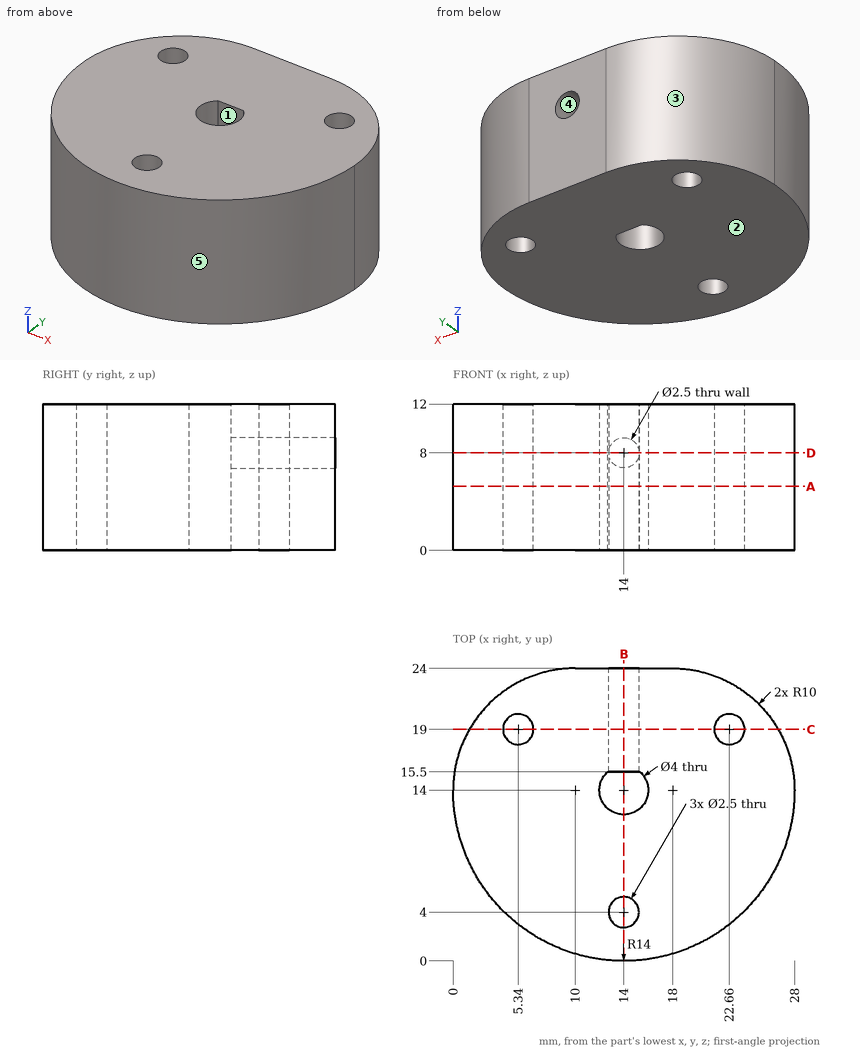
The drawing under review shows one solid part. Ordinate dimensions are in mm from its lowest x, y, z. A direction names the side the tool comes from. Give positions to 0.01 mm unless a question says otherwise; leave off trailing zeros. Order: outer loops, then holes, each group sorted by start corner. A loop starts at its lowest first (then second) coordinate and runs counter-clockwise, first axis right, second up. Notation, with made-up numbers: M 82.25,68 L 107.25,68 A22 cw 107.25,96 Z; hole C -8,32 d5. An arc over 180 degrees is marked long. Answer in a Markdown table with one row per item. Add a question column.
1. Machinability: for the marked faces 4 and 5, which of the approach directions +Z, -Z, +X, -X, +Y, -Y give a long, thin tool a straight path to every point of the face, cutting with its end or side? Answer none if there is none.
2. To check wall thickness, follow line 1 along X through (y, z) = (18, 3.5) (1 decimal); line 2 along Z through (x, y) = (14, 18); line 3 along Y through (x, z) = (4.5, 7) (1 decimal). State the ranges of each line that lie inside material, in increasing order.
3. Add section A-A on z = 5.25. State the section outline as (x, y) points, plus the area to 3 significant figures.
4. Add section C-C on y = 19. State the section outline as (x, z) points, plus the area to 3 significant figures.
5. Add section D-D on z = 8. State the section outline as (x, y) points.
6. For pin 1 Ø1.5 at (x, z) = (22, 7.5) entering from -Y; pin 2 Ø6 at (x, z) = (5.5, 8) entering from -Y (1 decimal); pin 3 Ø2 at (y, z) = (19, 3.5) entering from +X (1 decimal), all flat-tipped, find the tip position at first contact; note any pin that passes through.
7. Add section B-B on x = 14. State the section outline as (y, z) points.
8. Mouldability with a two-part tool opening along Y and no side actions: class the marked faces 1, 2 and 3 as released by +Y, released by -Y, zero draft, split by the parting line, or undercut.
The answers:
| question | item | result |
|---|---|---|
| 1 | face 4 | +Y |
| 1 | face 5 | +Z, -Z, -Y |
| 2 | line 1 | 0.8 to 4.6, 6.1 to 21.9, 23.4 to 27.2 |
| 2 | line 2 | 0 to 6.75, 9.25 to 12 |
| 2 | line 3 | 3.7 to 18.1, 19.9 to 22.4 |
| 3 | outline | M 0,14 A14 ccw 28,14 A10 ccw 18,24 L 10,24 A10 ccw Z; hole C 5.34,19 d2.5; hole M 12.68,15.5 A2 ccw long 15.32,15.5 Z; hole C 14,4 d2.5; hole C 22.66,19 d2.5 |
| 3 | area | 519 mm2 |
| 4 | outline | M 1.34,0 L 4.09,0 L 4.09,12 L 1.34,12 Z; M 6.59,0 L 21.41,0 L 21.41,12 L 6.59,12 Z; M 23.91,0 L 26.66,0 L 26.66,12 L 23.91,12 Z; hole C 14,8 d2.5 |
| 4 | area | 239 mm2 |
| 5 | outline | M 0,14 A14 ccw 28,14 A10 ccw 18,24 L 15.25,24 L 15.25,15.5 L 15.32,15.5 A2 cw long 12.68,15.5 L 12.75,15.5 L 12.75,24 L 10,24 A10 ccw Z; hole C 5.34,19 d2.5; hole C 14,4 d2.5; hole C 22.66,19 d2.5 |
| 6 | pin 1 | y = 2.02 |
| 6 | pin 2 | y = 1.1 |
| 6 | pin 3 | x = 27.2 |
| 7 | outline | M 0,0 L 2.75,0 L 2.75,12 L 0,12 Z; M 5.25,0 L 12,0 L 12,12 L 5.25,12 Z; M 15.5,0 L 24,0 L 24,6.75 L 15.5,6.75 Z; M 15.5,9.25 L 24,9.25 L 24,12 L 15.5,12 Z |
| 8 | face 1 | undercut |
| 8 | face 2 | zero draft |
| 8 | face 3 | released by +Y |
